The listing builds one solid part. Answer for the finished solid, in the listing's coordinates (mm). Round coordinates to 2 decimals unless told otherwise and drop trailing zeros. Write each loop counter-clockwise with the first axis right and the second up, starting at its lowest first coordinate (ties: lowest second). Pieces come first, ordered by that corner, then holes. Notation, with made-up numbers: M 42,30.25 L 56,30.25 A20 cw 56,34.25 Z; hole C 64.5,-29.5 d8. An arc over 180 degrees is marked long. Put each result on its own line as item: value. Start each with the question number.
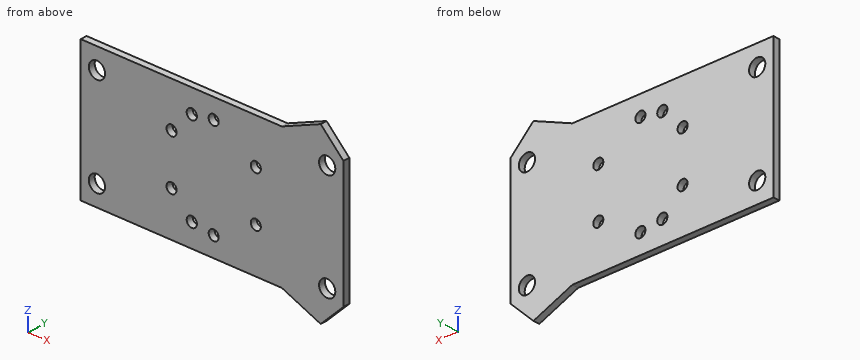
```python
from build123d import *
from build123d.topology import SkipClean

# Parameters (mm, degrees)
SKETCH_1_R          = 25
SKETCH_1_W          = 81
SKETCH_1_H          = 42
SKETCH_1_R_2        = 2.5
EXTRUDE_1_DEPTH     = 5
SKETCH_3_W          = 8.1
SKETCH_3_H          = 6.6
SKETCH_3_R          = 1.575
CUT_EXTRUDE_1_DEPTH = 2
SKETCH_3_2_R        = 1.575
CUT_EXTRUDE_2_DEPTH = 49.280430818
SKETCH_4_W          = 8
SKETCH_4_H          = 2.9
EXTRUDE_2_DEPTH     = 42
SKETCH_1_3_R        = 2.5
CUT_EXTRUDE_3_DEPTH = 42
EXTRUDE_START       = 21
SKETCH_5_W          = 11
SKETCH_5_H          = 2.9
EXTRUDE_3_DEPTH     = 5
SKETCH_5_W_2        = 12
EXTRUDE_3_2_DEPTH   = 5
CUT_EXTRUDE_4_REACH = 87.138
CHAMFER_1_SIZE      = 2
EXTRUDE_4_DEPTH     = 15
EXTRUDE_4_2_DEPTH   = 15
EXTRUDE_START_2     = -15
EXTRUDE_5_DEPTH     = 7.9
EXTRUDE_6_DEPTH     = 15
EXTRUDE_7_DEPTH     = 7.9
FILLET_1_R          = 5
SKETCH_12_R         = 2.5
SKETCH_12_R_2       = 1.575
EXTRUDE_8_DEPTH     = 2
SKETCH_13_W         = 180
SKETCH_13_H         = 120
CUT_EXTRUDE_5_DEPTH = 51.813384064
SKETCH_14_R         = 1.55
CUT_EXTRUDE_7_DEPTH = 10


# Read off the part's stored shape, not the designer's step: the extrude step
with BuildPart() as part:
    # Sketch 1 → Extrude 1 (new body)
    # profile 1 of 2: a face of its own
    with BuildSketch(Plane(origin=(0, 0, 0), x_dir=(1, 0, 0), z_dir=(0, 1, 0))):
        Circle(SKETCH_1_R)
    # profile 2 of 2: a face of its own
    with BuildSketch(Plane(origin=(0, 0, 0), x_dir=(1, 0, 0), z_dir=(0, 1, 0))):
        with Locations((-0.5, 0)):
            Rectangle(SKETCH_1_W, SKETCH_1_H)
        with Locations(Location((35, 16, 0), (0, 0, 270))):
            Circle(SKETCH_1_R_2, mode=Mode.SUBTRACT)
        with Locations(Location((35, -16, 0), (0, 0, 270))):
            Circle(SKETCH_1_R_2, mode=Mode.SUBTRACT)
        with Locations(Location((-36, 14.75, 0), (0, 0, 270))):
            Circle(SKETCH_1_R_2, mode=Mode.SUBTRACT)
        with Locations(Location((-36, -14.75, 0), (0, 0, 270))):
            Circle(SKETCH_1_R_2, mode=Mode.SUBTRACT)
    extrude(amount=EXTRUDE_1_DEPTH)

    # Sketch 3 → Cut-Extrude 1 (cut)
    # profile 1 of 2: a face of its own
    with BuildSketch(Plane(origin=(0, 5, 0), x_dir=(1, 0, 0), z_dir=(0, 1, 0))):
        with Locations((-6.75, -14)):
            Rectangle(SKETCH_3_W, SKETCH_3_H)
        with Locations(Location((-6.75, -14, 0), (0, 0, 90))):
            Circle(SKETCH_3_R, mode=Mode.SUBTRACT)
    # profile 2 of 2: a face of its own
    with BuildSketch(Plane(origin=(0, 5, 0), x_dir=(1, 0, 0), z_dir=(0, 1, 0))):
        with Locations((-6.75, 14)):
            Rectangle(SKETCH_3_W, SKETCH_3_H)
        with Locations(Location((-6.75, 14, 0), (0, 0, 270))):
            Circle(SKETCH_3_R, mode=Mode.SUBTRACT)
    extrude(amount=-CUT_EXTRUDE_1_DEPTH, mode=Mode.SUBTRACT)

    # Sketch 3_2 → Cut-Extrude 2 (cut, through all)
    with BuildSketch(Plane(origin=(0, 5, 0), x_dir=(1, 0, 0), z_dir=(0, 1, 0))):
        with Locations(Location((-6.75, 14, 0), (0, 0, 270))):
            Circle(SKETCH_3_2_R)
        with Locations(Location((-6.75, -14, 0), (0, 0, 270))):
            Circle(SKETCH_3_2_R)
    extrude(amount=-CUT_EXTRUDE_2_DEPTH, mode=Mode.SUBTRACT)

    # Sketch 4 → Extrude 2 (add)
    with BuildSketch(Plane.XY.offset(21)):
        with Locations((36, 6.45)):
            Rectangle(SKETCH_4_W, SKETCH_4_H)
        with Locations((-37, 6.45)):
            Rectangle(SKETCH_4_W, SKETCH_4_H)
    extrude(amount=-EXTRUDE_2_DEPTH)

    # Sketch 1_3 → Cut-Extrude 3 (cut)
    with BuildSketch(Plane(origin=(0, 0, 0), x_dir=(1, 0, 0), z_dir=(0, 1, 0))):
        with Locations(Location((35, 16, 0), (0, 0, 270))):
            Circle(SKETCH_1_3_R)
        with Locations(Location((35, -16, 0), (0, 0, 270))):
            Circle(SKETCH_1_3_R)
        with Locations(Location((-36, 14.75, 0), (0, 0, 180))):
            Circle(SKETCH_1_3_R)
        with Locations(Location((-36, -14.75, 0), (0, 0, 180))):
            Circle(SKETCH_1_3_R)
    extrude(amount=CUT_EXTRUDE_3_DEPTH, mode=Mode.SUBTRACT)


with BuildPart() as body_2:
    # Sketch 5 → Extrude 3 (new body)
    with BuildSketch(Plane.XY.offset(EXTRUDE_START)):
        with Locations((26.5, 6.45)):
            Rectangle(SKETCH_5_W, SKETCH_5_H)
    extrude_3 = extrude(amount=-EXTRUDE_3_DEPTH)


with BuildPart() as body_3:
    # Sketch 5 → Extrude 3 2 (new body)
    with BuildSketch(Plane.XY.offset(EXTRUDE_START)):
        with Locations((-27, 6.45)):
            Rectangle(SKETCH_5_W_2, SKETCH_5_H)
    extrude_3_2 = extrude(amount=-EXTRUDE_3_2_DEPTH)



with BuildPart() as part_1:
    add(part.part)

    # Mirror 2: Extrude 3, Extrude 3 2 across plane
    add(extrude_3.mirror(Plane(origin=(0, 0, 0), x_dir=(1, 0, 0), z_dir=(0, 0, -1))))
    add(extrude_3_2.mirror(Plane(origin=(0, 0, 0), x_dir=(1, 0, 0), z_dir=(0, 0, -1))))

    # Cut-Extrude 4: up to this face of the body (flat: up to its plane)
    cut_extrude_4_end = Plane(part_1.part.faces().sort_by_distance((32, 6.45, 2.5))[0])
    # Sketch 6 → Cut-Extrude 4 (cut, up to the picked face)
    with BuildSketch(Plane.ZY.offset(41), mode=Mode.PRIVATE) as cut_extrude_4_sk1:
        with BuildLine():
            Line((11.041960784, 8.971428571), (-11.041960784, 8.971428571))
            ThreePointArc((-11.041960784, 8.971428571), (-8.690257734, 7.239234925), (-6.072727273, 5.943265655))
            ThreePointArc((-6.072727273, 5.943265655), (0, 4.8), (6.072727273, 5.943265655))
            ThreePointArc((6.072727273, 5.943265655), (8.690257734, 7.239234925), (11.041960784, 8.971428571))
        make_face()
    cut_extrude_4_tool1 = split(extrude(cut_extrude_4_sk1.sketch, amount=-CUT_EXTRUDE_4_REACH, mode=Mode.PRIVATE), bisect_by=cut_extrude_4_end, keep=Keep.BOTH, mode=Mode.PRIVATE)
    add(cut_extrude_4_tool1.solids().sort_by(Axis((-41, 7.283597, 0), (1, 0, 0)))[0], mode=Mode.SUBTRACT)

    # Chamfer 1
    chamfer_1_edges = [part_1.edges().sort_by_distance(p)[0] for p in [
        (-41, 3.95, 21),
        (-41, 3.95, -21),
        (40, 3.95, -21),
        (40, 3.95, 21),
    ]]
    chamfer(chamfer_1_edges, length=CHAMFER_1_SIZE)



with BuildPart() as body_4:
    # Sketch 9 → Extrude 4 (new body)
    with BuildSketch(Plane.XZ):
        with BuildLine():
            Line((33, 26), (23.72846392, 26))
            ThreePointArc((23.72846392, 26), (24.88485791, 24.895458357), (25.989891949, 23.739534884))
            ThreePointArc((25.989891949, 23.739534884), (27.687521221, 22.340851231), (29.708138181, 21.471732017))
            ThreePointArc((29.708138181, 21.471732017), (30.719571772, 21.268231436), (31.749015733, 21.2))
            Line((31.749015733, 21.2), (37.8, 21.2))
            Line((37.8, 21.2), (33, 26))
        make_face()
    extrude(amount=-EXTRUDE_4_DEPTH)


with BuildPart() as body_5:
    # Sketch 9 → Extrude 4 2 (new body)
    with BuildSketch(Plane.XZ):
        with BuildLine():
            Line((33, -26), (37.8, -21.2))
            Line((37.8, -21.2), (31.749015733, -21.2))
            ThreePointArc((31.749015733, -21.2), (30.719571772, -21.268231436), (29.708138181, -21.471732017))
            ThreePointArc((29.708138181, -21.471732017), (27.687521221, -22.340851231), (25.989891949, -23.739534884))
            ThreePointArc((25.989891949, -23.739534884), (24.88485791, -24.895458357), (23.72846392, -26))
            Line((23.72846392, -26), (33, -26))
        make_face()
    extrude(amount=-EXTRUDE_4_2_DEPTH)


with BuildPart() as part_2:
    add(part_1.part)

    add(body_4.part)  # Extrude 5 merges body 4
    # Sketch 10 → Extrude 5 (add)
    with BuildSketch(Plane(origin=(0, 15, 0), x_dir=(1, 0, 0), z_dir=(0, 1, 0)).offset(EXTRUDE_START_2)):
        with BuildLine():
            Line((21, -21), (23.72846392, -26))
            ThreePointArc((23.72846392, -26), (24.88485791, -24.895458357), (25.989891949, -23.739534884))
            ThreePointArc((25.989891949, -23.739534884), (28.601924052, -21.863066908), (31.749015733, -21.2))
            Line((31.749015733, -21.2), (37.8, -21.2))
            Line((37.8, -21.2), (38, -21))
            Line((38, -21), (32, -21))
            Line((32, -21), (21, -21))
        make_face()
    extrude_5 = extrude(amount=EXTRUDE_5_DEPTH)


with BuildPart() as body_3_1:
    add(body_3.part)

    add(part_2.part)  # Extrude 6 merges part
    # Sketch 11 → Extrude 6 (add)
    with BuildSketch(Plane.XZ.offset(EXTRUDE_START_2)):
        with BuildLine():
            Line((-41, 23), (-41, 20.45))
            Line((-41, 20.45), (-40.520827978, 20.45))
            ThreePointArc((-40.520827978, 20.45), (-40.024975712, 20.455165886), (-39.5293387, 20.4706613))
            Line((-39.5293387, 20.4706613), (-39, 21))
            Line((-39, 21), (-35.43383476, 21))
            ThreePointArc((-35.43383476, 21), (-31.171725667, 22.363148102), (-27.240108871, 24.5))
            Line((-27.240108871, 24.5), (-41, 24.5))
            Line((-41, 24.5), (-41, 23))
        make_face()
        with BuildLine():
            Line((-39, 21), (-39.5293387, 20.4706613))
            ThreePointArc((-39.5293387, 20.4706613), (-39.301113021, 20.481274846), (-39.072999743, 20.494078772))
            ThreePointArc((-39.072999743, 20.494078772), (-38.358018151, 20.54847571), (-37.644999743, 20.624386527))
            ThreePointArc((-37.644999743, 20.624386527), (-36.534990206, 20.786132091), (-35.43383476, 21))
            Line((-35.43383476, 21), (-39, 21))
        make_face()
    extrude_6 = extrude(amount=EXTRUDE_6_DEPTH)

    # Extrude 7 outline → Extrude 7 (add)
    with BuildSketch(Plane(origin=(0, 0, 0), x_dir=(1, 0, 0), z_dir=(0, 1, 0))):
        with BuildLine():
            Line((-39.5293387, -20.4706613), (-41, -19))
            Line((-41, -19), (-41, -20.45))
            Line((-41, -20.45), (-40.520827978, -20.45))
            ThreePointArc((-40.520827978, -20.45), (-40.024975712, -20.455165886), (-39.5293387, -20.4706613))
        make_face()
        with BuildLine():
            Line((-21, -21), (-35.43383476, -21))
            ThreePointArc((-35.43383476, -21), (-31.171725667, -22.363148102), (-27.240108871, -24.5))
            Line((-27.240108871, -24.5), (-21, -21))
        make_face()
    extrude_7 = extrude(amount=EXTRUDE_7_DEPTH)

    # Mirror 3: Extrude 5, Extrude 6, Extrude 7 across plane
    add(extrude_5.mirror(Plane(origin=(0, 0, 0), x_dir=(1, 0, 0), z_dir=(0, 0, -1))))
    add(extrude_6.mirror(Plane(origin=(0, 0, 0), x_dir=(1, 0, 0), z_dir=(0, 0, -1))))
    add(extrude_7.mirror(Plane(origin=(0, 0, 0), x_dir=(1, 0, 0), z_dir=(0, 0, -1))))


with BuildPart() as body_2_1:
    add(body_2.part)

    # Combine 1: union body 3, body 5
    add(body_3_1.part)
    add(body_5.part)

    # Fillet 1
    fillet_1_edges = [body_2_1.edges().sort_by_distance(p)[0] for p in [
        (32, 6.45, 16),
        (-33, 6.45, 16),
        (-33, 6.45, -16),
        (32, 6.45, -16),
    ]]
    fillet(fillet_1_edges, radius=FILLET_1_R)

    # Sketch 12 → Extrude 8 (add)
    with SkipClean():  # the faces are left unmerged after this step: merging them gives an invalid solid
        with BuildSketch(Plane.XZ):
            Polygon((13.564659966, 21), (-13.564659966, 21), (-21, 21), (-41, 21), (-41, -21), (-21, -21), (-13.564659966, -21), (13.564659966, -21), (21, -21), (33, -26), (40, -19), (40, 19), (33, 26), (21, 21), align=None)
            with Locations((-36, -14.75)):
                Circle(SKETCH_12_R, mode=Mode.SUBTRACT)
            with Locations((-6.75, -14)):
                Circle(SKETCH_12_R_2, mode=Mode.SUBTRACT)
            with Locations((35, -16)):
                Circle(SKETCH_12_R, mode=Mode.SUBTRACT)
            with Locations((-36, 14.75)):
                Circle(SKETCH_12_R, mode=Mode.SUBTRACT)
            with Locations((-6.75, 14)):
                Circle(SKETCH_12_R_2, mode=Mode.SUBTRACT)
            with Locations((35, 16)):
                Circle(SKETCH_12_R, mode=Mode.SUBTRACT)
        extrude(amount=EXTRUDE_8_DEPTH)

    # Sketch 13 → Cut-Extrude 5 (cut, through all)
    with BuildSketch(Plane.XZ):
        with Locations((-41, 24.5)):
            Rectangle(SKETCH_13_W, SKETCH_13_H)
    extrude(amount=-CUT_EXTRUDE_5_DEPTH, mode=Mode.SUBTRACT)

    # Sketch 14 → Cut-Extrude 7 (cut)
    with BuildSketch(Plane.XZ):
        with Locations(Location((12.990381057, 7.5, 0), (0, 0, 270))):
            Circle(SKETCH_14_R)
        with Locations(Location((12.990381057, -7.5, 0), (0, 0, 270))):
            Circle(SKETCH_14_R)
        with Locations(Location((0, -15, 0), (0, 0, 270))):
            Circle(SKETCH_14_R)
        with Locations(Location((-12.990381057, -7.5, 0), (0, 0, 270))):
            Circle(SKETCH_14_R)
        with Locations(Location((-12.990381057, 7.5, 0), (0, 0, 270))):
            Circle(SKETCH_14_R)
        with Locations(Location((0, 15, 0), (0, 0, 270))):
            Circle(SKETCH_14_R)
    extrude(amount=CUT_EXTRUDE_7_DEPTH, mode=Mode.SUBTRACT)


solid = body_2_1.part
```
Item 1: Section C-C (y = -0.7) is taken. Count the separate pieces of the cut face and the enclosed holes in it, and give its area (3 significant figures).
Item 2: A flat-ended cylindrical pin translates along its axis: pin 1 (1 mm diameter, centred on x = 5, y = -1, fed in from -Z). Find the tip coordinate at first contact, or state that the pin passes through.
Item 3: Section B-B (z = 7.5) is taken. Give the vertices of the cut face in (x, y).
Item 4: Section D-D (x = -27) is taken. Give the vertices of the cut face in (y, z), and give its area (3 significant figures).
Item 5: Consider line 1 along Z through (x, y) = (0, -0.95); line 2 along Z through (x, y) = (-36, -0.45); line 3 along X through (y, z) = (-1, 7.5). Determine where each line is inside the solid, lowest interval first. Write a range as [from, to].
Item 6: Section A-A (x = 0) is taken. Give the vertices of the cut face in (y, z), and give its area (3 significant figures).
Output values:
1. separate pieces: 1
1. enclosed holes: 12
1. area: 3,340 mm^2
2. pin 1: stops at z = -21
3. outline: M -41,-2 L -14.54,-2 L -14.54,0 L -41,0 Z; M -11.44,-2 L 11.44,-2 L 11.44,0 L -11.44,0 Z; M 14.54,-2 L 40,-2 L 40,0 L 14.54,0 Z
4. outline: M -2,-21 L 0,-21 L 0,21 L -2,21 Z
4. area: 84.0 mm^2
5. line 1: z = [-21, -16.55], [-13.45, 13.45], [16.55, 21]
5. line 2: z = [-21, -17.25], [-12.25, 12.25], [17.25, 21]
5. line 3: x = [-41, -14.54], [-11.44, 11.44], [14.54, 40]
6. outline: M -2,-21 L 0,-21 L 0,-16.55 L -2,-16.55 Z; M -2,-13.45 L 0,-13.45 L 0,13.45 L -2,13.45 Z; M -2,16.55 L 0,16.55 L 0,21 L -2,21 Z
6. area: 71.6 mm^2
